Input: part model. Units: mm. Frame: model coordinates. Give positions to 0.01 mm unless a question says otherwise; leave off trailing zeros. Order: outer loops, then holes, each group sorted by start corner. A loop starts at its lowest first (then second) coordinate and runs counter-clockwise, first axis right, second up. Notation, with made-up numbers: (70, 19.25) - (75, 19.25) arc R14 cw to (75, 37.25) - close; hole circle Ø9 at (31, 26.5). An arc over 180 degrees is marked (long way). Answer in a Markdown table with one row per item. Add a question column.
1. Section query C-C on z = 5.75. Return loops of the section in (x, y).
2. Contact query for flat-ended pins moving along their axis: pin 1 (4 mm diameter, centred on x = 15, z = 1.5, fed in from -Y); pin 2 (1 mm diameter, centred on y = 18.5, z = 2, fed in from +X); pin 3 (6 mm diameter, centred on y = -13.5, z = 6, fed in from -X); pin 4 (7 mm diameter, centred on x = 0, y = 0, fed in from +Z). Output: stop coordinate, or through.
3. Ray query, line 1 (Y direction, x = 0, z = 4.5); line 2 (X direction, y = 13.5, z = 6.75); line 3 (X direction, y = -16, z = 7.25). Return the intervals inside material, ascending. Write a range as [from, to].
4. Section query A-A on y = 0. Return loops of the section in (x, z).
```python
from build123d import *

# Parameters (mm, degrees)
F0_R     = 24.5
F0_R_2   = 4
F1_DEPTH = 10
F2_R     = 3
F3_R     = 2


with BuildPart() as f1:
    # F0 (on Top) → F1 (new body)
    with BuildSketch(Plane.XY):
        Circle(F0_R)
        Circle(F0_R_2, mode=Mode.SUBTRACT)
    extrude(amount=F1_DEPTH)

    # F2
    f2_edges = [f1.edges().sort_by_distance(p)[0] for p in [
        (-24.5, 0, 10),
        (-4, 0, 10),
    ]]
    fillet(f2_edges, radius=F2_R)

    # F3
    f3_edges = [f1.edges().sort_by_distance(p)[0] for p in [
        (-24.5, 0, 0),
    ]]
    fillet(f3_edges, radius=F3_R)


solid = f1.part
```
Answer:
| question | item | result |
|---|---|---|
| 1 | outline | circle Ø49 at (0, 0); hole circle Ø8 at (0, 0) |
| 2 | pin 1 | stops at y = -20.74 |
| 2 | pin 2 | stops at x = 16.62 |
| 2 | pin 3 | stops at x = -22.14 |
| 2 | pin 4 | passes through |
| 3 | line 1 | y = [-24.5, -4], [4, 24.5] |
| 3 | line 2 | x = [-20.45, 20.45] |
| 3 | line 3 | x = [-18.54, 18.54] |
| 4 | outline | (-24.5, 2) arc R2 ccw to (-22.5, 0) - (-4, 0) - (-4, 7) arc R3 ccw to (-7, 10) - (-21.5, 10) arc R3 ccw to (-24.5, 7) - close; (4, 0) - (22.5, 0) arc R2 ccw to (24.5, 2) - (24.5, 7) arc R3 ccw to (21.5, 10) - (7, 10) arc R3 ccw to (4, 7) - close |
